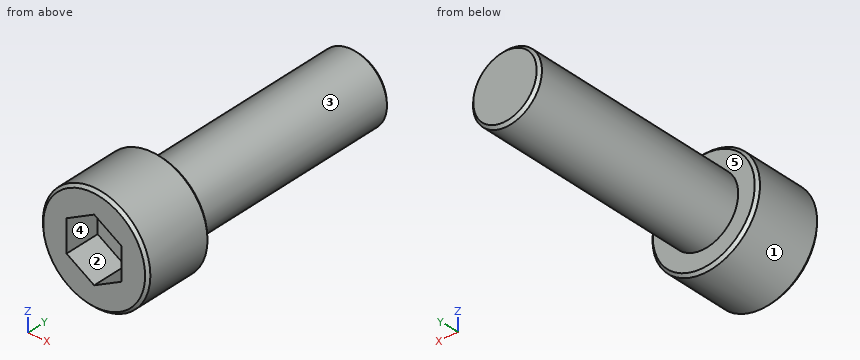
```python
from build123d import *

# Parameters (mm, degrees)
SKETCH_1_R          = 1.95
SKETCH_1_R_2        = 1.25
EXTRUDE_1_DEPTH     = 2.5
SKETCH_1_3_R        = 1.25
EXTRUDE_2_DEPTH     = 8
CUT_EXTRUDE_START   = -1.25
CUT_EXTRUDE_1_DEPTH = 2.25
CHAMFER_1_SIZE      = 0.1


with BuildPart() as part:
    # Sketch 1 → Extrude 1 (new body)
    with BuildSketch(Plane(origin=(0, 0, 0), x_dir=(1, 0, 0), z_dir=(0, 1, 0))):
        Circle(SKETCH_1_R)
        Circle(SKETCH_1_R_2, mode=Mode.SUBTRACT)
        Circle(SKETCH_1_R_2)
        Polygon((1, 0.577350269), (0, 1.154700538), (-1, 0.577350269), (-1, -0.577350269), (0, -1.154700538), (1, -0.577350269), align=None, mode=Mode.SUBTRACT)
        Polygon((1, -0.577350269), (1, 0.577350269), (0, 1.154700538), (-1, 0.577350269), (-1, -0.577350269), (0, -1.154700538), align=None)
    extrude(amount=-EXTRUDE_1_DEPTH)

    # Sketch 1_3 → Extrude 2 (add)
    with BuildSketch(Plane(origin=(0, 0, 0), x_dir=(1, 0, 0), z_dir=(0, 1, 0))):
        Circle(SKETCH_1_3_R)
        Polygon((1, 0.577350269), (0, 1.154700538), (-1, 0.577350269), (-1, -0.577350269), (0, -1.154700538), (1, -0.577350269), align=None, mode=Mode.SUBTRACT)
        Polygon((1, -0.577350269), (1, 0.577350269), (0, 1.154700538), (-1, 0.577350269), (-1, -0.577350269), (0, -1.154700538), align=None)
    extrude(amount=EXTRUDE_2_DEPTH)

    # Sketch 1_6 → Cut-Extrude 1 (cut, through all)
    with BuildSketch(Plane(origin=(0, 0, 0), x_dir=(1, 0, 0), z_dir=(0, 1, 0)).offset(CUT_EXTRUDE_START)):
        Polygon((0, 1.154700538), (-1, 0.577350269), (-1, -0.577350269), (0, -1.154700538), (1, -0.577350269), (1, 0.577350269), align=None)
    extrude(amount=-CUT_EXTRUDE_1_DEPTH, mode=Mode.SUBTRACT)

    # Chamfer 1
    chamfer_1_edges = [part.edges().sort_by_distance(p)[0] for p in [
        (-1.95, 0, 0),
        (-1.95, -2.5, 0),
        (-1.25, 8, 0),
    ]]
    chamfer(chamfer_1_edges, length=CHAMFER_1_SIZE)


solid = part.part
```
Input: part model. Units: mm. Frame: model coordinates. Face numbers are marked on the shaded views. A direction names the side the tool comes from. Give positions to 0.01 mm unless a question says otherwise; leave off trailing zeros. Order: outer loops, then holes, each group sorted by start corner. A loop starts at its lowest first (then second) coordinate and runs counter-clockwise, first axis right, second up. Notation, with made-up numbers: (69, -22) - (91, -22) arc R21 ccw to (91, 12) - close; hole circle Ø2 at (74.5, 79.5). An arc over 180 degrees is marked (long way). One line per item, written item: value.
1. Cut plane C-C, the plane y = -0.75. Output: boundary loops of the cut face in (x, z), and give its area (3 significant figures).
Determined:
outline: circle Ø3.9 at (0, 0)
area: 11.9 mm2
2. Draft query along Z for the marked faces 3, 4 and 5. Return one class per face: released by +Z, released by -Z, zero draft, split by the parting line, or undercut.
Determined:
face 3: split by the parting line
face 4: undercut
face 5: zero draft
3. Cut plane A-A, the plane z = 0. Output: boundary loops of the cut face in (x, y).
Determined:
outline: (-1.95, -2.4) - (-1.85, -2.5) - (-1, -2.5) - (-1, -1.25) - (1, -1.25) - (1, -2.5) - (1.85, -2.5) - (1.95, -2.4) - (1.95, -0.1) - (1.85, 0) - (1.25, 0) - (1.25, 7.9) - (1.15, 8) - (-1.15, 8) - (-1.25, 7.9) - (-1.25, 0) - (-1.85, 0) - (-1.95, -0.1) - close
4. Reachability of the marked faces 1 and 2 from +Z, -Z, +X, -X, +Y, -Y: full face, straight path, thin tool, end or side. Return the list, or none.
Determined:
face 1: +Y, -Y
face 2: -Y
5. Cut plane B-B, the plane y = 4. Output: boundary loops of the cut face in (x, z), and give its area (3 significant figures).
Determined:
outline: circle Ø2.5 at (0, 0)
area: 4.91 mm2
6. Pin query (flat end, axial travel): pin 1 Ø2 at (x, z) = (0.5, 0) entering from -Y. Return the tip coordinate at first contact, or that it passes through.
Determined:
pin 1: y = -2.5
7. Line query: probe 1 along Z at (x, y) = (0, 0.75); probe 2 along Y at (x, z) = (0.45, 0.8); probe 3 along Y at (x, z) = (0.5, -1.35). Output: solid intervals per line, ascending.
Determined:
probe 1: -1.25 to 1.25
probe 2: -1.25 to 8
probe 3: -2.5 to 0
